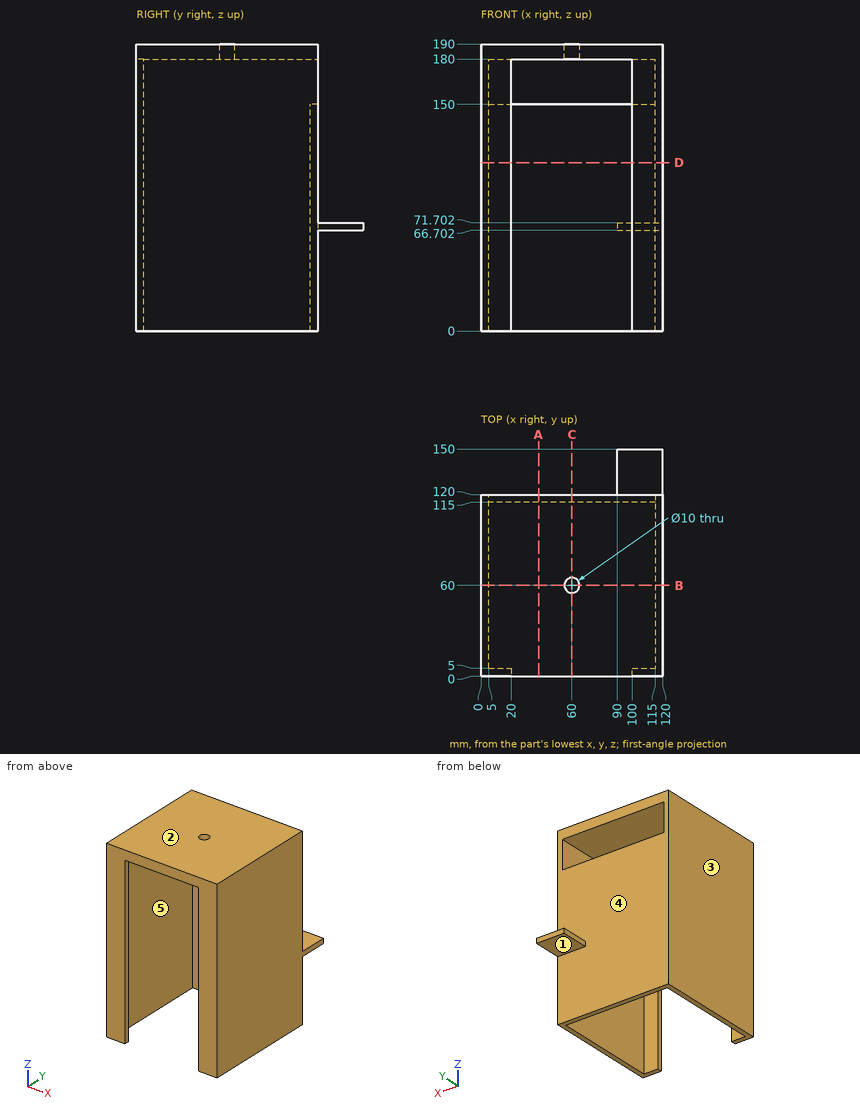
Part print with two shaded views. Sizes in mm from the minimum x, y, z corner. A direction names the side the tool comes from. Round coordinates to 2 decimals unless told otherwise and drop trailing zeros. Order: outer loops, then holes, each group sorted by start corner. A loop starts at its lowest first (then second) coordinate and runs counter-clockwise, first axis right, second up. Notation, with made-up numbers: (-26, 31) - (-10, 31) arc R14 cw to (-10, 50) - close; hole circle Ø5 at (36.5, -36.75). An arc over 180 degrees is marked (long way). Answer in a Markdown table with one row per item. Add a question column.
(1) Drop flat-ended pins along their axis: pin 1 Ø3 at (x, y) = (49.5, 67.5) entering from -Z; pin 2 Ø5 at (x, z) = (52.5, 35) entering from +Y; pin 3 Ø9 at (x, y) = (110.5, 135.5) entering from +Z; pin 4 Ø12 at (y, z) = (128.5, 51) entering from +X. Give the stop position or say it passes through.
(2) Band-saw the part on A-A on x = 38. List the corners of the cut face in (y, z).
(3) Band-saw the part on C-C on x = 60. List the corners of the cut face in (y, z).
(4) Probe L1, parallel to X at y = 23, z = 73; L2, parallel to Y at x = 60, z = 186.5. List the from-to ranges inside material, lowest first. Write a range as [from, to].
(5) Band-saw the part on B-B on y = 60. List the corners of the cut face in (x, z), and give its area (3 significant figures).
(6) 3-axis set-ups, long thin cutter, end or side, ignore diameter. For the marked faces 1 and 2: which of +Z, -Z, +X, -X, +Y, -Y reach the whole face in a straight line?
(7) Mould opens along X. For the marked faces 3, 4 and 5 say: +X half, -X half, draft (parallel to the pull), parting line (faces both ways), or undercut.
(8) Band-saw the part on D-D on z = 111.5. List the corners of the cut face in (x, y), and give its area (3 significant figures).
Data:
| question | item | result |
|---|---|---|
| 1 | pin 1 | stops at z = 180 |
| 1 | pin 2 | stops at y = 120 |
| 1 | pin 3 | stops at z = 71.7 |
| 1 | pin 4 | passes through |
| 2 | outline | (0, 180) - (120, 180) - (120, 190) - (0, 190) - close; (115, 0) - (120, 0) - (120, 150) - (115, 150) - close |
| 3 | outline | (0, 180) - (55, 180) - (55, 190) - (0, 190) - close; (65, 180) - (120, 180) - (120, 190) - (65, 190) - close; (115, 0) - (120, 0) - (120, 150) - (115, 150) - close |
| 4 | L1 | x = [0, 5], [115, 120] |
| 4 | L2 | y = [0, 55], [65, 120] |
| 5 | outline | (0, 0) - (5, 0) - (5, 180) - (55, 180) - (55, 190) - (0, 190) - close; (65, 180) - (115, 180) - (115, 0) - (120, 0) - (120, 190) - (65, 190) - close |
| 5 | area | 2,900 mm^2 |
| 6 | face 1 | -Z, +X, -X, +Y |
| 6 | face 2 | +Z, +X, -X, +Y, -Y |
| 7 | face 3 | -X half |
| 7 | face 4 | draft |
| 7 | face 5 | undercut |
| 8 | outline | (0, 0) - (20, 0) - (20, 5) - (5, 5) - (5, 115) - (115, 115) - (115, 5) - (100, 5) - (100, 0) - (120, 0) - (120, 120) - (0, 120) - close |
| 8 | area | 1,900 mm^2 |
